```python
from build123d import *

# Parameters (mm, degrees)
CUT_EXTRUDE_START   = -4.0000001
CUT_EXTRUDE_1_DEPTH = 3.921539232
FILLET_1_R          = 0.4


with BuildPart() as part:
    # Эскиз1 → Повернуть1 (revolve)
    with BuildSketch(Plane(origin=(0, 0, 0), x_dir=(0, 0, -1), z_dir=(1, 0, 0))):
        with BuildLine():
            Line((16, 0), (16, 2.4))
            Line((16, 2.4), (14.4, 4))
            Line((14.4, 4), (1.02, 4))
            ThreePointArc((1.02, 4), (0.957844465, 4.004858646), (0.897198888, 4.019316553))
            Line((0.897198888, 4.019316553), (0.277198888, 4.219316553))
            ThreePointArc((0.277198888, 4.219316553), (0.076642269, 4.36454347), (0, 4.6))
            Line((0, 4.6), (0, 6.5))
            Line((0, 6.5), (-8, 6.5))
            Line((-8, 6.5), (-8, 3.6))
            Line((-8, 3.6), (-7.653589838, 3))
            Line((-7.653589838, 3), (-4, 3))
            Line((-4, 3), (-2.267949192, 0))
            Line((-2.267949192, 0), (16, 0))
        make_face()
    revolve(axis=Axis((0, 0, -16), (0, 0, 1)))

    # Вырез-Вытянуть1: read off the stored shape, not the designer's step
    # Вырез-Вытянуть1 outline → Вырез-Вытянуть1 (cut)
    with BuildSketch(Plane.XY.offset(8).offset(CUT_EXTRUDE_START)):
        with BuildLine():
            Line((3, 0), (3, 1.732050808))
            Line((3, 1.732050808), (1.499999997, 2.598076213))
            ThreePointArc((1.499999997, 2.598076213), (2.59807621, 1.500000002), (3, 0))
        make_face()
        with BuildLine():
            ThreePointArc((-1.499999956, 2.598076237), (2.4e-08, 3), (1.499999997, 2.598076213))
            Line((1.499999997, 2.598076213), (0, 3.464101615))
            Line((0, 3.464101615), (-1.499999956, 2.598076237))
        make_face()
        with BuildLine():
            Line((3, -1.732050808), (3, 0))
            ThreePointArc((3, 0), (2.59807621, -1.500000002), (1.499999997, -2.598076213))
            Line((1.499999997, -2.598076213), (3, -1.732050808))
        make_face()
        with BuildLine():
            ThreePointArc((-3, 0), (-2.598076199, 1.500000022), (-1.499999956, 2.598076237))
            Line((-1.499999956, 2.598076237), (-3, 1.732050808))
            Line((-3, 1.732050808), (-3, 0))
        make_face()
        with BuildLine():
            Line((0, -3.464101615), (1.499999997, -2.598076213))
            ThreePointArc((1.499999997, -2.598076213), (0, -3), (-1.499999997, -2.598076213))
            Line((-1.499999997, -2.598076213), (0, -3.464101615))
        make_face()
        with BuildLine():
            ThreePointArc((-1.499999997, -2.598076213), (-2.59807621, -1.500000002), (-3, 0))
            Line((-3, 0), (-3, -1.732050808))
            Line((-3, -1.732050808), (-1.499999997, -2.598076213))
        make_face()
    extrude(amount=CUT_EXTRUDE_1_DEPTH, mode=Mode.SUBTRACT)

    # Cut-Extrude 1 2 outline → Cut-Extrude 1 2 (revolve)
    with BuildSketch(Plane.XZ):
        Polygon((3.464101616, 4.267949193), (2.999999957, 3.999999975), (3.464101615, 3.9999999), align=None)
    revolve(axis=Axis((0, 0, 0), (0, 0, 1)))

    # Скругление1
    fillet_1_edges = [part.edges().sort_by_distance(p)[0] for p in [
        (0, -6.5, 0),
        (0, -6.5, 8),
    ]]
    fillet(fillet_1_edges, radius=FILLET_1_R)


solid = part.part
```
Source: CAD feature listing. Evaluate the final solid. Frame: model axes, mm. A direction names the side the tool comes from. Coordinates: 2 decimals unless noted, no trailing zeros. Loops run counter-clockwise (first coordinate to the right, second up) from the corner with the lowest first, then second, coordinate; pieces in that order, holes last. Notation, with made-up numbers: (39.5, 52) - (46.5, 52) arc R18 ccw to (46.5, 60) - close; hole circle Ø11 at (44, 75). An arc over 180 degrees is marked (long way). Answer as CSV lines item,"result".
1. Ray query, line 1 (X direction, y = 0, z = 5); line 2 (X direction, y = 1, z = 4); line 3 (Z direction, x = 4, y = -4.5). Return the intervals inside material, ascending.
Established:
line 1,"x = -6.5 to -3, 3 to 6.5"
line 2,"x = -6.42 to -2.83, 2.83 to 6.42"
line 3,"z = 0 to 8"
2. Contact query for flat-ended pins moving along their axis: pin 1 (3 mm diameter, centred on y = -4, z = -8.5, fed in from +X); pin 2 (5 mm diameter, centred on y = 2, z = -4.5, fed in from +X); pin 3 (2 mm diameter, centred on y = 4, z = -12.5, fed in from +X). Output: stop coordinate, or through.
Established:
pin 1,"stops at x = 3.12"
pin 2,"stops at x = 4"
pin 3,"stops at x = 2.65"
3. Section A-A (z = -1.75). Return loops of the section in (x, y).
Established:
outline,"circle Ø8 at (0, 0)"
4. Mould query, pull axis Y, two halves, no side actions, for faces 4 (the flat face through (0, 0, -16)), 5 (the cylindrical face through (3.955, -5.158, 4.05)), 6 (the flat face through (-3, 0, 6)). Classes: released by +Y, released by -Y, zero draft, split by the parting line, or undercut.
Established:
face 4,"zero draft"
face 5,"split by the parting line"
face 6,"undercut"
5. Reachability of faces 1 (the flat face through (-5, -1, 0)), 2 (the flat face through (3, 0, 6)), 3 (the flat face through (3, 3, 8)) from +Z, -Z, +X, -X, +Y, -Y: full face, straight path, thin tool, end or side. Return the list, or none.
Established:
face 1,"-Z"
face 2,"+Z"
face 3,"+Z, +X, -X, +Y, -Y"
